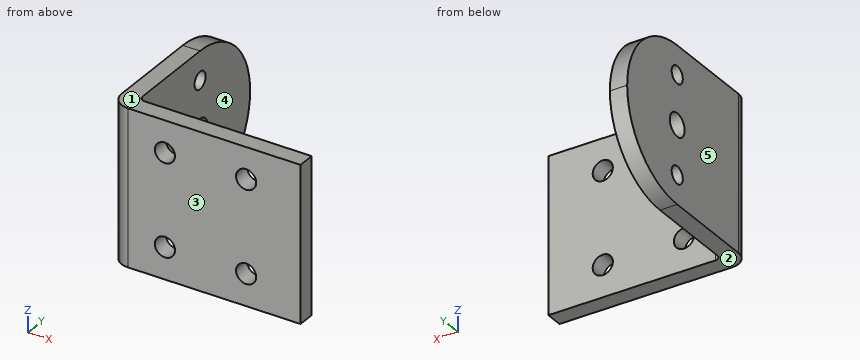
from build123d import *

# Parameters (mm, degrees)
P_IDAT_VYSUNUT_M1_DEPTH  = 27
ZAOBLIT1_R               = 1
SKICA2_R                 = 1.75
ODEBRAT_VYSUNUT_M1_DEPTH = 3
ZAOBLIT2_R               = 3
ODEBRAT_VYSUNUT_M2_DEPTH = 3
SKICA3_3_R               = 1.5
ODEBRAT_VYSUNUT_M3_DEPTH = 3
SKICA3_4_R               = 2
ODEBRAT_VYSUNUT_M4_DEPTH = 3


with BuildPart() as part:
    # Skica1 → P_idat vysunut_m1 (new body)
    with BuildSketch(Plane.XY):
        Polygon((0, 0), (0, 33), (3, 33), (3, 3), (33, 3), (33, 0), align=None)
    extrude(amount=P_IDAT_VYSUNUT_M1_DEPTH)

    # Zaoblit1
    zaoblit1_edges = [part.edges().sort_by_distance(p)[0] for p in [
        (3, 3, 13.5),
    ]]
    fillet(zaoblit1_edges, radius=ZAOBLIT1_R)

    # Skica2 → Odebrat vysunut_m1 (cut)
    with BuildSketch(Plane.XZ):
        with Locations((9.45, 21.5)):
            Circle(SKICA2_R)
        with Locations((23.55, 21.5)):
            Circle(SKICA2_R)
        with Locations(Location((23.55, 5.5, 0), (0, 0, 180))):
            Circle(SKICA2_R)
        with Locations(Location((9.45, 5.5, 0), (0, 0, 180))):
            Circle(SKICA2_R)
    extrude(amount=-ODEBRAT_VYSUNUT_M1_DEPTH, mode=Mode.SUBTRACT)

    # Zaoblit2
    zaoblit2_edges = [part.edges().sort_by_distance(p)[0] for p in [
        (0, 0, 13.5),
    ]]
    fillet(zaoblit2_edges, radius=ZAOBLIT2_R)

    # Skica3 → Odebrat vysunut_m2 (cut)
    with BuildSketch(Plane.ZY):
        with BuildLine():
            Line((27, 33), (13.5, 33))
            ThreePointArc((13.5, 33), (23.045941546, 29.045941546), (27, 19.5))
            Line((27, 19.5), (27, 33))
        make_face()
        with BuildLine():
            Line((0, 33), (0, 19.5))
            ThreePointArc((0, 19.5), (3.954058454, 29.045941546), (13.5, 33))
            Line((13.5, 33), (0, 33))
        make_face()
    extrude(amount=-ODEBRAT_VYSUNUT_M2_DEPTH, mode=Mode.SUBTRACT)

    # Skica3_3 → Odebrat vysunut_m3 (cut)
    with BuildSketch(Plane.ZY):
        with Locations((5, 19.5)):
            Circle(SKICA3_3_R)
        with Locations((22, 19.5)):
            Circle(SKICA3_3_R)
    extrude(amount=-ODEBRAT_VYSUNUT_M3_DEPTH, mode=Mode.SUBTRACT)

    # Skica3_4 → Odebrat vysunut_m4 (cut)
    with BuildSketch(Plane.ZY):
        with Locations((13.5, 19.5)):
            Circle(SKICA3_4_R)
    extrude(amount=-ODEBRAT_VYSUNUT_M4_DEPTH, mode=Mode.SUBTRACT)


solid = part.part
Could you check a few things on this model? Use its own coordinates, in mm. Face numbers are marked on the shaded views. A direction names the side the tool comes from. Give positions to 0.01 mm unless a question says otherwise; leave off trailing zeros. Order: outer loops, then holes, each group sorted by start corner. A loop starts at its lowest first (then second) coordinate and runs counter-clockwise, first axis right, second up. Notation, with made-up numbers: M 68.5,-27.75 L 85.5,-27.75 A20 ccw 85.5,-2.75 Z; hole C -16.75,32.5 d5. An arc over 180 degrees is marked long. One line per question, with ' | ' between items.
1. I want a section at A-A (x = 9.45). List the corners of the cut face in (y, z) for me, and give its area (3 significant figures).
Results:
outline: M 0,0 L 3,0 L 3,3.75 L 0,3.75 Z; M 0,7.25 L 3,7.25 L 3,19.75 L 0,19.75 Z; M 0,23.25 L 3,23.25 L 3,27 L 0,27 Z | area: 60.0 mm²
2. If I drill on line 1 (Z direction, x = 23.55, y = 1); line 2 (X direction, y = 12, z = 16.25), over which ranges is the centre line in solid material (lowest first)?
Results:
line 1: 0 to 3.75, 7.25 to 19.75, 23.25 to 27 | line 2: 0 to 3
3. I'm going to push flat-ended pins straight in: pin 1 (6 mm diameter, centred on x = 5, y = 24, fed in from -Z); pin 2 (2 mm diameter, centred on y = 16, z = 14.5, fed in from +X); pin 3 (3 mm diameter, centred on x = 9.45, z = 21.5, fed in from -Y); pin 4 (10 mm diameter, centred on x = 20, z = 10.5, fed in from +Y). Where does each tip first touch, or does it pass through?
Results:
pin 1: z = 0.19 | pin 2: x = 3 | pin 3: through | pin 4: y = 3
4. I want a section at B-B (z = 22). List the corners of the cut face in (x, y) for me, and give its area (3 significant figures).
Results:
outline: M 0,3 A3 ccw 3,0 L 7.77,0 L 7.77,3 L 4,3 A1 cw 3,4 L 3,18 L 0,18 Z; M 0,21 L 3,21 L 3,29.99 L 0,29.99 Z; M 11.13,0 L 21.87,0 L 21.87,3 L 11.13,3 Z; M 25.23,0 L 33,0 L 33,3 L 25.23,3 Z | area: 149 mm²
5. I want a section at D-D (z = 14). List the corners of the cut face in (x, y) for me, and give its area (3 significant figures).
Results:
outline: M 0,3 A3 ccw 3,0 L 33,0 L 33,3 L 4,3 A1 cw 3,4 L 3,17.56 L 0,17.56 Z; M 0,21.44 L 3,21.44 L 3,32.99 L 0,32.99 Z | area: 176 mm²
6. For the marked faces 4 and 5, which set-ups out of +Z, -Z, +X, -X, +Y, -Y let a thin tool reach every point of the face, with its end or its side?
Results:
face 4: +Z, -Z, +X, +Y | face 5: +Z, -Z, -X, +Y, -Y
7. I want a section at C-C (y = 20). List the corners of the cut face in (x, z) for me.
Results:
outline: M 0,0.01 L 3,0.01 L 3,3.59 L 0,3.59 Z; M 0,6.41 L 3,6.41 L 3,11.56 L 0,11.56 Z; M 0,15.44 L 3,15.44 L 3,20.59 L 0,20.59 Z; M 0,23.41 L 3,23.41 L 3,26.99 L 0,26.99 Z
8. We'd pull the mould along Z, two halves only. Please class the marked faces 1, 2 and 3: +Z half, -Z half, draft (parallel to the pull), parting line (faces both ways), or undercut.
Results:
face 1: +Z half | face 2: -Z half | face 3: draft
